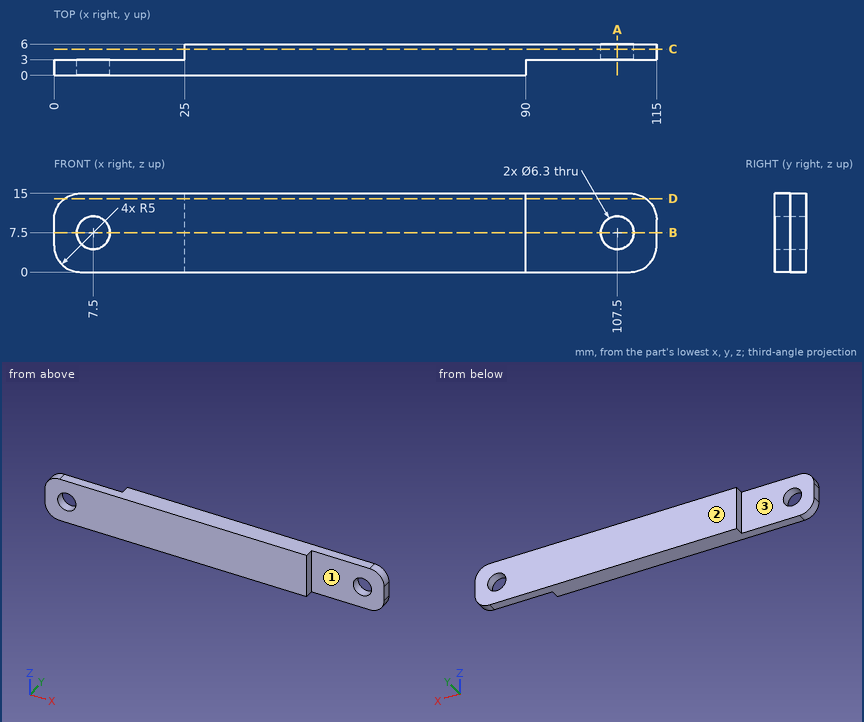
Verification items for this drawing (mm, ordinates from the low corner). A direction names the side the tool comes from. Give positions to 0.01 mm unless a question says otherwise; leave off trailing zeros. Loops run counter-clockwise (first coordinate to the right, second up) from the corner with the lowest first, then second, coordinate; pieces in that order, holes last. Notation, with made-up numbers: M 3.25,-2.5 L 15.25,-2.5 A11 cw 15.25,14.5 Z; hole C 21.25,-10.5 d1. An arc over 180 degrees is marked long. Write item = value, one per line. Start each with the question number.
1. Section check B-B, the plane z = 7.5. Enter the section's corners in (x, y).
2. Section check A-A, the plane x = 107.5. Enter the section's corners in (y, z), plus the area to 3 significant figures.
3. Section check C-C, the plane y = 5. Enter the section's corners in (x, z).
4. Thickness scan on probe 1 along Z at (x, y) = (7.5, 2.4); probe 2 along X at (y, z) = (4.35, 7.5); probe 3 along X at (y, z) = (0.95, 7.5). Record the ranges inside material, lowest first.
5. Section check D-D, the plane z = 14. Enter the section's corners in (x, y).
6. Tool access check on the marked faces 1, 2 and 3. Record the directions out of +Z, -Z, +X, -X, +Y, -Y that give a thin tool (end or side, any length) a straight path to the whole face; none if there is none.
7. Go/stop test with flat-tipped pins: P1, Ø0.9, axis at y = 4.5, z = 9, coming from the -X side; P2, Ø1, axis at y = 2.5, z = 11, coming from the -X side; P3, Ø5.5, axis at x = 7.5, z = 7.5, coming from the +Y side. Record where each tip stops, or that it passes through.
Values follow:
q1.outline = M 0,0 L 4.35,0 L 4.35,3 L 0,3 Z; M 10.65,0 L 90,0 L 90,3 L 104.35,3 L 104.35,6 L 25,6 L 25,3 L 10.65,3 Z; M 110.65,3 L 115,3 L 115,6 L 110.65,6 Z
q2.outline = M 3,0 L 6,0 L 6,4.35 L 3,4.35 Z; M 3,10.65 L 6,10.65 L 6,15 L 3,15 Z
q2.area = 26.1 mm^2
q3.outline = M 25,0 L 110,0 A5 ccw 115,5 L 115,10 A5 ccw 110,15 L 25,15 Z; hole C 107.5,7.5 d6.3
q4.probe_1 = 0 to 4.35, 10.65 to 15
q4.probe_2 = 25 to 104.35, 110.65 to 115
q4.probe_3 = 0 to 4.35, 10.65 to 90
q5.outline = M 2,0 L 90,0 L 90,3 L 113,3 L 113,6 L 25,6 L 25,3 L 2,3 Z
q6.face_1 = +Z, -Z, +X, -Y
q6.face_2 = +Z, -Z, +X, -X, +Y
q6.face_3 = +Z, -Z, -X, +Y
q7.P1 = 25
q7.P2 = 0.03
q7.P3 = through
